```python
from build123d import *

# Parameters (mm, degrees)
SKETCH_1_R      = 6
EXTRUDE_1_DEPTH = 38
SKETCH_2_R      = 8
EXTRUDE_2_DEPTH = 8
SKETCH_4_R      = 6
EXTRUDE_3_DEPTH = 12
SKETCH_5_R      = 5
EXTRUDE_4_DEPTH = 12


with BuildPart() as part:
    # 草图1 → 凸台-拉伸1 (new body)
    with BuildSketch(Plane(origin=(0, 0, 0), x_dir=(1, 0, 0), z_dir=(0, 1, 0))):
        with Locations(Location((0, 0, 0), (0, 0, 270))):
            Circle(SKETCH_1_R)
    extrude(amount=EXTRUDE_1_DEPTH)

    # 草图2 → 凸台-拉伸2 (add)
    with BuildSketch(Plane(origin=(0, 38, 0), x_dir=(1, 0, 0), z_dir=(0, 1, 0))):
        with Locations(Location((0, 0, 0), (0, 0, 270))):
            Circle(SKETCH_2_R)
    extrude(amount=EXTRUDE_2_DEPTH)

    # 草图4 → 凸台-拉伸3 (add)
    with BuildSketch(Plane(origin=(0, 46, 0), x_dir=(1, 0, 0), z_dir=(0, 1, 0))):
        with Locations(Location((0, 0, 0), (0, 0, 270))):
            Circle(SKETCH_4_R)
    extrude(amount=EXTRUDE_3_DEPTH)

    # 草图5 → 凸台-拉伸4 (add)
    with BuildSketch(Plane(origin=(0, 58, 0), x_dir=(1, 0, 0), z_dir=(0, 1, 0))):
        with Locations(Location((0, 0, 0), (0, 0, 270))):
            Circle(SKETCH_5_R)
    extrude(amount=EXTRUDE_4_DEPTH)


solid = part.part
```
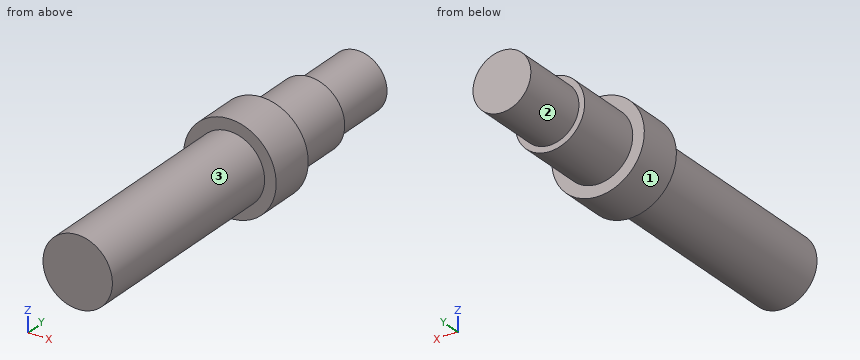
Geometry: final body of the model. Coordinates: model frame, mm. Face numbers are marked on the shaded views. A direction names the side the tool comes from. Coordinates: 2 decimals unless noted, no trailing zeros. Order: outer loops, then holes, each group sorted by start corner. A loop starts at its lowest first (then second) coordinate and runs counter-clockwise, first axis right, second up. Notation, with made-up numbers: M 62,-12 L 116,-12 A21 cw 116,19 Z; hole C 14.25,62.5 d8. An arc over 180 degrees is marked long. Answer as CSV lines item,"result".
Q1. Line query: probe 1 along Y at (x, z) = (-1, -5.5); probe 2 along Y at (x, z) = (5.75, -5.5); probe 3 along X at (y, z) = (39, 7.25). Output: solid intervals per line, ascending. Write a range as [from, to].
Answers:
probe 1,"y = [0, 58]"
probe 2,"y = [38, 46]"
probe 3,"x = [-3.38, 3.38]"
Q2. Section D-D on y = 39. Return the cut outline in (x, z).
Answers:
outline,"C 0,0 d16"
Q3. Section A-A on z = 0. Return the cut outline in (x, y), and give its area (3 significant figures).
Answers:
outline,"M -8,38 L -6,38 L -6,0 L 6,0 L 6,38 L 8,38 L 8,46 L 6,46 L 6,58 L 5,58 L 5,70 L -5,70 L -5,58 L -6,58 L -6,46 L -8,46 Z"
area,"848 mm^2"
Q4. First-contact query: P1, Ø4, axis at x = -4.5, y = 44.5, coming from the +Z side; P2, Ø1, axis at x = 2.5, y = 58, coming from the +Z side; P3, Ø2, axis at y = 13, z = 5.5, coming from the -X side. Flat tips, straight axial feed; report the tip coordinate or a pass-through.
Answers:
P1,"stops at z = 7.6"
P2,"stops at z = 5.66"
P3,"stops at x = -3.97"
Q5. Set-up query: the marked faces 1, 2 and 3. Return all of +Z, -Z, +X, -X, +Y, -Y with unobstructed straight access to the full face (end or side cutting, diameter ignored); none if empty.
Answers:
face 1,"+Y, -Y"
face 2,"+Y"
face 3,"-Y"
Q6. Section C-C on y = 50.5. Return the cut outline in (x, z).
Answers:
outline,"C 0,0 d12"
Q7. Section B-B on x = 0. Return the cut outline in (y, z).
Answers:
outline,"M 0,-6 L 38,-6 L 38,-8 L 46,-8 L 46,-6 L 58,-6 L 58,-5 L 70,-5 L 70,5 L 58,5 L 58,6 L 46,6 L 46,8 L 38,8 L 38,6 L 0,6 Z"
